Here's how the part is built. I have some questions about the finished solid (model axes, mm). Coordinates: 2 decimals unless noted, no trailing zeros. Order: outer loops, then holes, each group sorted by start corner. A loop starts at its lowest first (then second) coordinate and runs counter-clockwise, first axis right, second up. Notation, with made-up numbers: (59.5, -5.5) - (99.5, -5.5) arc R11 ccw to (99.5, 14.5) - close; hole circle Ø2 at (64.25, 11.25). An arc over 180 degrees is marked (long way). Answer as CSV lines item,"result". Start each with the question number.
Q1. Thinking about a two-plate mould opening in Z: for faces 1 (the face through (5, 0, 72)), 2 (the face through (0, 0, 104)), 3 (the face through (0, 0, 0)), 4 (the face through (-2.146, -4.125, 40.993)), which applies, released by +Z, released by -Z, zero draft, split by the parting line, or undercut?
Q2. I need wall thicknesses on line 1 (X direction, y = 0.25, z = 50); line 2 (Z direction, x = 4.5, y = 2); line 3 (Z direction, x = 2.25, y = 4.25). Which ranges of each line are inside material? Lowest first, please.
Q3. Suppose I cut it at A-A (z = 45.5). Please give me the cut outline in (x, y).
Q4. For pin 1 Ø6 at (y, z) = (4, 34.5) entering from -X; pin 2 Ø1.5 at (y, z) = (3, 74) entering from +X; pin 3 Ø1 at (y, z) = (-2, 32) entering from -X, each with a flat end and sliding along its axis, tell me the tip position at first contact or that it passes through.
from build123d import *

# Parameters (mm, degrees)
SKETCH_1_R      = 5
EXTRUDE_1_DEPTH = 104
SKETCH_2_W      = 3.498862739
SKETCH_2_H      = 1
CHAMFER_1_SIZE  = 0.5


with BuildPart() as part:
    # 草图1 → 拉伸1 (new body)
    with BuildSketch(Plane.XY):
        with Locations(Location((0, 0, 0), (0, 0, 180))):
            Circle(SKETCH_1_R)
    extrude(amount=EXTRUDE_1_DEPTH)

    # 草图2 → 切除-旋转1 (revolve, cut)
    with BuildSketch(Plane(origin=(0, 0, 0), x_dir=(1, 0, 0), z_dir=(0, 1, 0)), mode=Mode.PRIVATE) as cut_revolve_1_sk:
        with Locations((6.39943137, -41)):
            Rectangle(SKETCH_2_W, SKETCH_2_H)
    revolve(cut_revolve_1_sk.sketch.rotate(Axis((0, 0, 104), (0, 0, -1)), 180), axis=Axis((0, 0, 104), (0, 0, -1)), mode=Mode.SUBTRACT)

    # 倒角1
    chamfer_1_edges = [part.edges().sort_by_distance(p)[0] for p in [
        (5, 0, 0),
        (5, 0, 104),
    ]]
    chamfer(chamfer_1_edges, length=CHAMFER_1_SIZE)


solid = part.part
Here are the results:
1,face 1,"zero draft"
1,face 2,"released by +Z"
1,face 3,"released by -Z"
1,face 4,"undercut"
2,line 1,"x = -4.99 to 4.99"
2,line 2,"z = 0.42 to 40.5, 41.5 to 103.58"
2,line 3,"z = 0.31 to 40.5, 41.5 to 103.69"
3,outline,"circle Ø10 at (0, 0)"
4,pin 1,"stops at x = -4.9"
4,pin 2,"stops at x = 4.47"
4,pin 3,"stops at x = -4.77"
